from build123d import *

# Parameters (mm, degrees)
SKETCH1_R           = 19.05
SKETCH1_R_2         = 2.413
BOSS_EXTRUDE1_DEPTH = 3.175


with BuildPart() as part:
    # Sketch1 → Boss-Extrude1 (new body)
    with BuildSketch(Plane(origin=(0, 0, 0), x_dir=(1, 0, 0), z_dir=(0, 1, 0))):
        Circle(SKETCH1_R)
        with Locations((0, 12.7)):
            Circle(SKETCH1_R_2, mode=Mode.SUBTRACT)
        with Locations((12.7, 0)):
            Circle(SKETCH1_R_2, mode=Mode.SUBTRACT)
        with Locations((0, -12.7)):
            Circle(SKETCH1_R_2, mode=Mode.SUBTRACT)
        with Locations((-12.7, 0)):
            Circle(SKETCH1_R_2, mode=Mode.SUBTRACT)
        Polygon((-7.332348419, 0), (-3.666174209, -6.35), (3.666174209, -6.35), (7.332348419, 0), (3.666174209, 6.35), (-3.666174209, 6.35), align=None, mode=Mode.SUBTRACT)
    extrude(amount=BOSS_EXTRUDE1_DEPTH)


solid = part.part
CAD build for the part. Positions are in the model's coordinates, mm. A direction names the side the tool comes from. Give positions to 0.01 mm unless a question says otherwise; leave off trailing zeros. Write each loop counter-clockwise with the first axis right and the second up, starting at its lowest first coordinate (ties: lowest second). Pieces come first, ordered by that corner, then holes. Notation, with made-up numbers: (35, 56.25) -> (80, 56.25) arc R16 ccw to (80, 68.25) -> close; hole circle Ø4 at (80, 54). An arc over 180 degrees is marked (long way). Return JSON: item names as keys, results as strings.
Item 1: Band-saw the part on D-D (x = -12.7). List the corners of the cut face in (y, z) (3 decimals), then the cut area to 3 significant figures.
Answer below:
{"outline": "(0, -14.199) -> (3.175, -14.199) -> (3.175, -2.413) -> (0, -2.413) -> close; (0, 2.413) -> (3.175, 2.413) -> (3.175, 14.199) -> (0, 14.199) -> close", "area": "74.8 mm2"}
Item 2: Drop flat-ended pins along their axis: pin 1 (1 mm diameter, centred on x = -0.5, y = 1.5, fed in from -Z); pin 2 (1 mm diameter, centred on x = 0.5, y = 1.5, fed in from +Z); pin 3 (3 mm diameter, centred on x = 12.7, z = 0, fed in from -Y); pin 4 (1 mm diameter, centred on y = 0.5, z = 13.5, fed in from +X). Give the stop position or say it passes through.
Answer below:
{"pin 1": "stops at z = -19.05", "pin 2": "stops at z = 19.05", "pin 3": "passes through", "pin 4": "stops at x = 13.92"}
Item 3: Band-saw the part on B-B (z = -14.5). List the corners of the cut face in (x, y) (3 decimals), then the cut area to 3 significant figures.
Answer below:
{"outline": "(-12.355, 0) -> (-1.607, 0) -> (-1.607, 3.175) -> (-12.355, 3.175) -> close; (1.607, 0) -> (12.355, 0) -> (12.355, 3.175) -> (1.607, 3.175) -> close", "area": "68.3 mm2"}
Item 4: Band-saw the part on C-C (y = 2). List the corners of the cut face in (x, z), then the cut area to 3 significant figures.
Answer below:
{"outline": "circle Ø38.1 at (0, 0); hole circle Ø4.83 at (-12.7, 0); hole (-7.33, 0) -> (-3.67, -6.35) -> (3.67, -6.35) -> (7.33, 0) -> (3.67, 6.35) -> (-3.67, 6.35) -> close; hole circle Ø4.83 at (0, -12.7); hole circle Ø4.83 at (0, 12.7); hole circle Ø4.83 at (12.7, 0)", "area": "927 mm2"}
Item 5: Drill centre lines: probe 1 along X at (y, z) = (1.4, 0); probe 2 along Z at (x, y) = (0, 0.75); probe 3 along X at (y, z) = (0.65, 2). Where is each one in solid material? Low to high.
Answer below:
{"probe 1": "x = -19.05 to -15.11, -10.29 to -7.33, 7.33 to 10.29, 15.11 to 19.05", "probe 2": "z = -19.05 to -15.11, -10.29 to -6.35, 6.35 to 10.29, 15.11 to 19.05", "probe 3": "x = -18.94 to -14.05, -11.35 to -6.18, 6.18 to 11.35, 14.05 to 18.94"}
Item 6: Band-saw the part on A-A (x = 0). List the corners of the cut face in (y, z) (3 decimals), then the cut area to 3 significant figures.
Answer below:
{"outline": "(0, -19.05) -> (3.175, -19.05) -> (3.175, -15.113) -> (0, -15.113) -> close; (0, -10.287) -> (3.175, -10.287) -> (3.175, -6.35) -> (0, -6.35) -> close; (0, 6.35) -> (3.175, 6.35) -> (3.175, 10.287) -> (0, 10.287) -> close; (0, 15.113) -> (3.175, 15.113) -> (3.175, 19.05) -> (0, 19.05) -> close", "area": "50.0 mm2"}
Item 7: Tool access for faces 4 (the flat face through (8, 0, 0)), 5 (the flat face through (5.474, 1.565, 3.219)): list every direction of +Z, -Z, +X, -X, +Y, -Y with a clear straight run to the whole face (end or side of a thin tool).
Answer below:
{"face 4": "+Z, -Z, +X, -X, -Y", "face 5": "+Y, -Y"}
Item 8: Two-plate mould, pull along X, no slides. Class faces 1 (the cylindrical face through (10.29, 1.57, -0.11)), 2 (the flat face through (8, 3.175, 0)), 3 (the cylindrical face through (-15.12, 1.57, 11.59)): +X half, -X half, draft (parallel to the pull), parting line (faces both ways), or undercut.
Answer below:
{"face 1": "undercut", "face 2": "draft", "face 3": "parting line"}
